```python
from build123d import *

# Parameters (mm, degrees)
SKETCH1_W             = 30
SKETCH1_H             = 2
BOSS_EXTRUDE1_DEPTH   = 3.5
BOSS_EXTRUDE1_2_DEPTH = 3.5
SKETCH2_W             = 30
SKETCH2_H             = 19
BOSS_EXTRUDE2_DEPTH   = 2
SKETCH3_W             = 9
SKETCH3_H             = 8
BOSS_EXTRUDE3_DEPTH   = 4


with BuildPart() as part:
    # Sketch1 → Boss-Extrude1 (new body)
    with BuildSketch(Plane(origin=(0, 0, 0), x_dir=(1, 0, 0), z_dir=(0, 1, 0))):
        with Locations((15, -1)):
            Rectangle(SKETCH1_W, SKETCH1_H)
    extrude(amount=BOSS_EXTRUDE1_DEPTH)



with BuildPart() as body_2:
    # Sketch1 → Boss-Extrude1 2 (new body)
    with BuildSketch(Plane(origin=(0, 0, 0), x_dir=(1, 0, 0), z_dir=(0, 1, 0))):
        with Locations((15, -18)):
            Rectangle(SKETCH1_W, SKETCH1_H)
    extrude(amount=BOSS_EXTRUDE1_2_DEPTH)


with BuildPart() as part_1:
    add(part.part)

    add(body_2.part)  # Boss-Extrude2 merges body 2
    # Sketch2 → Boss-Extrude2 (add)
    with BuildSketch(Plane(origin=(0, 3.5, 0), x_dir=(1, 0, 0), z_dir=(0, 1, 0))):
        with Locations((15, -9.5)):
            Rectangle(SKETCH2_W, SKETCH2_H)
    extrude(amount=BOSS_EXTRUDE2_DEPTH)

    # Sketch3 → Boss-Extrude3 (add)
    with BuildSketch(Plane(origin=(0, 5.5, 0), x_dir=(1, 0, 0), z_dir=(0, 1, 0))):
        with Locations((-0.587922654, -9)):
            Rectangle(SKETCH3_W, SKETCH3_H)
    extrude(amount=BOSS_EXTRUDE3_DEPTH)


solid = part_1.part
```
Check sheet for the modelled part. Datum: model origin and axes. Units: mm. A direction names the side the tool comes from. Coordinates: 2 decimals unless noted, no trailing zeros. Write each loop counter-clockwise with the first axis right and the second up, starting at its lowest first coordinate (ties: lowest second). Pieces come first, ordered by that corner, then holes. Notation, with made-up numbers: (39.5, 48.5) - (44.5, 48.5) arc R26 cw to (44.5, 84.5) - close; hole circle Ø5 at (32.5, -38.75). An arc over 180 degrees is marked (long way). One line per question, with ' | ' between items.
Item 1: Gauge pin test, flat ends, axial feed: P1, Ø3, axis at y = 7.5, z = 10, coming from the +X side; P2, Ø1.2, axis at x = -3, y = 7, coming from the +Z side; P3, Ø4, axis at x = 13.5, z = 9.5, coming from the -Y side; P4, Ø2, axis at y = 8, z = 16.5, coming from the -X side. Record the tip position at first contact, or that the pin passes through.
Determined:
P1: stops at x = 3.91 | P2: stops at z = 13 | P3: stops at y = 3.5 | P4: passes through
Item 2: Sectioned sample at C-C on y = 6. Record the boundary of the cut face in (x, z), plus the area to 3 significant figures.
Determined:
outline: (-5.09, 5) - (3.91, 5) - (3.91, 13) - (-5.09, 13) - close | area: 72.0 mm2
Item 3: Access from +Z, -Z, +X, -X, +Y, -Y to the whole of each face (thin tool, end or side, straight path). Record for faces 4 (the face through (-1, 7, 13)), 5 (the face through (-3, 5.5, 9)), 6 (the face through (3.912, 7, 9)), 7 (the face through (-1, 7, 5)), 8 (the face through (15, 2, 2)).
Determined:
face 4: +Z, +X, -X, +Y | face 5: +Z, -Z, -X, -Y | face 6: +Z, -Z, +X, +Y | face 7: -Z, +X, -X, +Y | face 8: +X, -X, -Y
Item 4: Sectioned sample at D-D on x = 2.5. Record the boundary of the cut face in (y, z).
Determined:
outline: (0, 0) - (5.5, 0) - (5.5, 5) - (9.5, 5) - (9.5, 13) - (5.5, 13) - (5.5, 19) - (0, 19) - (0, 17) - (3.5, 17) - (3.5, 2) - (0, 2) - close
Item 5: Sectioned sample at B-B on z = 5.5. Record the boundary of the cut face in (x, y), plus the area to 3 significant figures.
Determined:
outline: (-5.09, 5.5) - (0, 5.5) - (0, 3.5) - (30, 3.5) - (30, 5.5) - (3.91, 5.5) - (3.91, 9.5) - (-5.09, 9.5) - close | area: 96.0 mm2
Item 6: Sectioned sample at A-A on x = 18. Record the boundary of the cut face in (y, z).
Determined:
outline: (0, 0) - (5.5, 0) - (5.5, 19) - (0, 19) - (0, 17) - (3.5, 17) - (3.5, 2) - (0, 2) - close
Item 7: Thickness scan on line 1 (Z direction, x = 28.5, y = 3); line 2 (Y direction, x = 4, z = 14.75); line 3 (Y direction, x = 9.5, z = 1). Record the ranges inside material, lowest first. Write a range as [from, to].
Determined:
line 1: z = [0, 2], [17, 19] | line 2: y = [3.5, 5.5] | line 3: y = [0, 5.5]
Item 8: Mould release check, pull along X, two halves, no side actions. Record for faces 1 (the face through (15, 3.5, 9)), 2 (the face through (30, 4, 10)), 3 (the face through (0, 4, 10)): pulls with the +X half, pulls with the -X half, needs draft (parallel to the pull), parting line crosses it, or undercut.
Determined:
face 1: needs draft | face 2: pulls with the +X half | face 3: pulls with the -X half
